from build123d import *


with BuildPart() as part:
    # Esquisse1 → Base-Révolution (revolve)
    with BuildSketch(Plane(origin=(0, 0, 0), x_dir=(1, 0, 0), z_dir=(0, 1, 0)), mode=Mode.PRIVATE) as base_r_volution_sk:
        with BuildLine():
            Line((0, 13.5725), (0, 20.523333333))
            ThreePointArc((0, 20.523333333), (0.139612434, 20.860387566), (0.476666667, 21))
            Line((0.476666667, 21), (6.673333333, 21))
            ThreePointArc((6.673333333, 21), (7.010387566, 20.860387566), (7.15, 20.523333333))
            Line((7.15, 20.523333333), (7.15, 19.9275))
            Line((7.15, 19.9275), (6.673333333, 19.9275))
            Line((6.673333333, 19.9275), (6.673333333, 20.6425))
            Line((6.673333333, 20.6425), (5.958333333, 20.6425))
            Line((5.958333333, 20.6425), (5.958333333, 20.285))
            Line((5.958333333, 20.285), (0.715, 20.285))
            Line((0.715, 20.285), (0.715, 15.208155728))
            Line((0.715, 15.208155728), (1.7875, 13.93))
            Line((1.7875, 13.93), (3.75375, 13.93))
            ThreePointArc((3.75375, 13.93), (4.199319064, 14.458527228), (4.795581349, 14.10875))
            Line((4.795581349, 14.10875), (5.3625, 14.10875))
            Line((5.3625, 14.10875), (5.3625, 13.5725))
            Line((5.3625, 13.5725), (4.29, 12.5))
            Line((4.29, 12.5), (2.325553645, 13.215))
            Line((2.325553645, 13.215), (1.253053645, 13.215))
            Line((1.253053645, 13.215), (0.400949826, 12.5))
            Line((0.400949826, 12.5), (0, 12.977833396))
            Line((0, 12.977833396), (0.292816141, 13.223535312))
            Line((0.292816141, 13.223535312), (0, 13.5725))
        make_face()
    revolve(base_r_volution_sk.sketch.rotate(Axis((0, 0, 0), (1, 0, 0)), 180), axis=Axis((0, 0, 0), (1, 0, 0)))


solid = part.part
Model file for the job. Use its own axes, mm. A direction names the side the tool comes from. Give positions to 0.01 mm unless a question says otherwise; leave off trailing zeros. Write item = value, one per line.
(1) Probe line 1 along Y through (x, z) = (2.1, 0) (3 decimals); line 2 along Z through (x, y) = (3.5, 3.5); line 3 along Y through (x, z) = (1.5, -8). List the from-to ranges inside material, lowest first.
Determined:
line_1 = -21 to -20.285, -13.93 to -13.215, 13.215 to 13.93, 20.285 to 21
line_2 = -20.71 to -19.98, -13.48 to -12.3, 12.3 to 13.48, 19.98 to 20.71
line_3 = -19.42 to -18.64, -11.82 to -10.52, 10.52 to 11.82, 18.64 to 19.42
(2) Flat gauge pins, fed straight in: P1, Ø1.5, axis at x = 4, y = -11.5, coming from the -Z side; P2, Ø12.5, axis at y = -2.5, z = -10, coming from the +X side; P3, Ø4, axis at x = 4, z = 3, coming from the +Y side. Where does each tip first touch, or does it go through?
Determined:
P1 = -18.04
P2 = 5.36
P3 = 20.98
(3) Mould opens along Z. For faces 4 (the face through (3.3, 12.34, -16.1)), 5 (the face through (3.62, -6.31, 20.03)), 6 (the face through (7.15, -17, -11)) say: released by +Z, released by -Z, zero draft, split by the parting line, or undercut.
Determined:
face_4 = undercut
face_5 = split by the parting line
face_6 = zero draft
(4) Tool access for faces 1 (the face through (6.31, -6.2, 19.69)), 2 (the face through (0, 13.4, -4.3)), 3 (the face through (6.91, -19.76, -2.59)): list every direction of +Z, -Z, +X, -X, +Y, -Y with a clear straight run to the whole face (end or side of a thin tool).
Determined:
face_1 = none
face_2 = +Z, -Z, -X, +Y, -Y
face_3 = +X
